```python
from build123d import *

# Parameters (mm, degrees)
F0_W     = 609.6
F0_H     = 914.4
F1_DEPTH = 1524
F2_T     = -6.35
F3_W     = 609.6
F3_H     = 1524
F3_W_2   = 406.4
F3_H_2   = 1320.8
F4_DEPTH = 6.35


with BuildPart() as f1:
    # F0 (on Top) → F1 (new body)
    with BuildSketch(Plane.XY):
        with Locations((-304.8, -457.2)):
            Rectangle(F0_W, F0_H)
    extrude(amount=F1_DEPTH)

    # F2
    f2_openings = [f1.faces().sort_by_distance(p)[0] for p in [
        (-304.8, -914.4, 762),
    ]]
    offset(amount=F2_T, openings=f2_openings)

    # F3 (on face) → F4 (join)
    with BuildSketch(Plane.XZ.offset(914.4)):
        with Locations((-304.8, 762)):
            Rectangle(F3_W, F3_H)
        with Locations((-304.8, 762)):
            Rectangle(F3_W_2, F3_H_2, mode=Mode.SUBTRACT)
    extrude(amount=-F4_DEPTH)


solid = f1.part
```
Check sheet for the modelled part. Datum: model origin and axes. Units: mm. A direction names the side the tool comes from. Round coordinates to 2 decimals unless told otherwise and drop trailing zeros. Order: outer loops, then holes, each group sorted by start corner. A loop starts at its lowest first (then second) coordinate and runs counter-clockwise, first axis right, second up. Notation, with made-up numbers: (-30.75, 54.5) -> (6.25, 54.5) arc R20 ccw to (6.25, 87.5) -> close; hole circle Ø10 at (-36, 9). An arc over 180 degrees is marked (long way). One line per item, written item: value. Start each with the question number.
Q1. Cross-section at B-B (x = -178.5). Record the boundary of the cut face in (y, z), and give its area (3 significant figures).
Q2. Cross-section at A-A (y = -331). Record the boundary of the cut face in (x, z).
Q3. Cross-section at C-C (x = -84.5). Record the boundary of the cut face in (y, z), and give its area (3 significant figures).
Q4. Mould release check, pull along Z, two halves, no side actions. Record for faces 3 (the face through (-309, -451, 0)), 4 (the face through (-309, -451, 6.35)), 5 (the face through (-6.35, -464, 751)), 6 (the face through (0, -464, 751)): pulls with the +Z half, pulls with the -Z half, needs draft (parallel to the pull), parting line crosses it, or undercut.
Q5. Gauge pin test, flat end, axial feed: pin 1 Ø2 at (x, z) = (-350, 480) entering from -Y. Record the tip position at first contact, or that the pin passes through.
Q6. Set-up check for faces 1 (the face through (-309, -6.35, 751)), 2 (the face through (-512, -914.4, 751)): record each of +Z, -Z, +X, -X, +Y, -Y from which the full face is reachable in a straight line by a thin tool's end or side.
Q7. Cross-section at D-D (z = 1380). Record the boundary of the cut face in (x, y).
Q8. Thickness scan on line 1 (Z direction, x = -36.5, y = -141); line 2 (X direction, y = -37.5, z = 255). Record the ranges inside material, lowest first.
Completed:
1. outline: (-914.4, 0) -> (0, 0) -> (0, 1524) -> (-914.4, 1524) -> (-914.4, 1422.4) -> (-908.05, 1422.4) -> (-908.05, 1517.65) -> (-6.35, 1517.65) -> (-6.35, 6.35) -> (-908.05, 6.35) -> (-908.05, 101.6) -> (-914.4, 101.6) -> close
1. area: 22,400 mm²
2. outline: (-609.6, 0) -> (0, 0) -> (0, 1524) -> (-609.6, 1524) -> close; hole (-603.25, 6.35) -> (-6.35, 6.35) -> (-6.35, 1517.65) -> (-603.25, 1517.65) -> close
3. outline: (-914.4, 0) -> (0, 0) -> (0, 1524) -> (-914.4, 1524) -> close; hole (-908.05, 6.35) -> (-6.35, 6.35) -> (-6.35, 1517.65) -> (-908.05, 1517.65) -> close
3. area: 30,800 mm²
4. face 3: pulls with the -Z half
4. face 4: undercut
4. face 5: undercut
4. face 6: needs draft
5. pin 1: stops at y = -6.35
6. face 1: none
6. face 2: +Z, -Z, +X, -X, -Y
7. outline: (-609.6, -914.4) -> (-508, -914.4) -> (-508, -908.05) -> (-603.25, -908.05) -> (-603.25, -6.35) -> (-6.35, -6.35) -> (-6.35, -908.05) -> (-101.6, -908.05) -> (-101.6, -914.4) -> (0, -914.4) -> (0, 0) -> (-609.6, 0) -> close
8. line 1: z = 0 to 6.35, 1517.65 to 1524
8. line 2: x = -609.6 to -603.25, -6.35 to 0
